Geometry: final body of the model. Coordinates: model frame, mm. A direction names the side the tool comes from. Give positions to 0.01 mm unless a question says otherwise; leave off trailing zeros. Loops run counter-clockwise (first coordinate to the right, second up) from the corner with the lowest first, then second, coordinate; pieces in that order, holes last. Notation, with made-up numbers: (68, 18.25) -> (98, 18.25) arc R17 cw to (98, 36.25) -> close; hole circle Ø9 at (-39.5, -22). An arc over 180 degrees is marked (long way). Answer in a Markdown table with one row per item. Add a question column.
1) Section query C-C (z = 4). Return the cut outline in (x, y).
2) Line query: line 1 (X direction, y = -16, z = 7); line 2 (X direction, y = -22.75, z = 27); line 3 (X direction, y = -2.75, z = 25.25). Output: solid intervals per line, ascending. Write a range as from..to.
3) Access query for faces 1 (the flat face through (-7, -10.414, 15)), 2 (the flat face through (49, -15.038, 15)), 3 (the flat face through (-18.668, -20, 15)), 4 (the flat face through (54, -12.5, 15)). Directions: +Z, -Z, +X, -X, +Y, -Y. A direction counts if a zero-diameter tool reaches every point of the face in a straight line with its end or side. Return the directions, or none.
4) First-contact query: P1, Ø15, axis at x = 24.5, z = 20.5, coming from the +Y side; P2, Ø10, axis at x = -12, z = 25, coming from the -Y side; P3, Ø3, axis at y = -4, z = 16.5, coming from the +X side. Flat tips, straight axial feed; report the tip coordinate or a pass-through.
5) Section query B-B (x = 49.5). Return the cut outline in (y, z).
6) Section query A-A (y = -16.75). Return the cut outline in (x, z).
7) Draft query along X for faces 5 (the flat face through (-28.375, -12, 15)), 6 (the flat face through (60.081, -19, 15)), 7 (the flat face through (5.6, -20, 15)), 8 (the flat face through (-23, 0, 15)). Return one class per face: +X half, -X half, draft (parallel to the pull), parting line (faces both ways), or undercut.
8) Section query D-D (y = -4.25). Return the cut outline in (x, z).
```python
from build123d import *

# Parameters (mm, degrees)
F0_W     = 24.2680183989
F0_H     = 5.0877342001
F0_W_2   = 35.3016227051
F0_H_2   = 3.6045075208
F0_W_3   = 2.852525562
F0_H_3   = 2.53832
F1_DEPTH = 30


with BuildPart() as f1:
    # F0 (on Top) → F1 (new body)
    with BuildSketch(Plane.XY):
        Polygon((-18.6677063226, -10.4143796489), (-18.6677063226, 0), (-28.3749136821, 0), (-28.3749136821, -25), (-18.6677063226, -25), (-18.6677063226, -15.5021138489), align=None)
        with Locations((-6.5336971231, -12.9582467489)):
            Rectangle(F0_W, F0_H)
        Polygon((5.6003120763, 0), (5.6003120763, -10.4143796489), (5.6003120763, -15.5021138489), (5.6003120763, -25), (15.563129677, -25), (15.563129677, -21.3954924792), (15.563129677, 0), align=None)
        with Locations((33.2139410295, -23.1977462396)):
            Rectangle(F0_W_2, F0_H_2)
        Polygon((50.864752382, -21.3954924792), (50.864752382, -25), (60.0811056793, -25), (60.0811056793, -12.5), (50.864752382, -12.5), (50.864752382, -15.03832), align=None)
        with Locations((49.438489601, -13.76916)):
            Rectangle(F0_W_3, F0_H_3)
    extrude(amount=F1_DEPTH)


solid = f1.part
```
Evaluation:
| question | item | result |
|---|---|---|
| 1 | outline | (-28.37, -25) -> (-18.67, -25) -> (-18.67, -15.5) -> (5.6, -15.5) -> (5.6, -25) -> (60.08, -25) -> (60.08, -12.5) -> (48.01, -12.5) -> (48.01, -15.04) -> (50.86, -15.04) -> (50.86, -21.4) -> (15.56, -21.4) -> (15.56, 0) -> (5.6, 0) -> (5.6, -10.41) -> (-18.67, -10.41) -> (-18.67, 0) -> (-28.37, 0) -> close |
| 2 | line 1 | -28.37..-18.67, 5.6..15.56, 50.86..60.08 |
| 2 | line 2 | -28.37..-18.67, 5.6..60.08 |
| 2 | line 3 | -28.37..-18.67, 5.6..15.56 |
| 3 | face 1 | +Z, -Z, +Y |
| 3 | face 2 | +Z, -Z |
| 3 | face 3 | +Z, -Z, -Y |
| 3 | face 4 | +Z, -Z, +X, +Y |
| 4 | P1 | y = -21.4 |
| 4 | P2 | y = -15.5 |
| 4 | P3 | x = 15.56 |
| 5 | outline | (-25, 0) -> (-21.4, 0) -> (-21.4, 30) -> (-25, 30) -> close; (-15.04, 0) -> (-12.5, 0) -> (-12.5, 30) -> (-15.04, 30) -> close |
| 6 | outline | (-28.37, 0) -> (-18.67, 0) -> (-18.67, 30) -> (-28.37, 30) -> close; (5.6, 0) -> (15.56, 0) -> (15.56, 30) -> (5.6, 30) -> close; (50.86, 0) -> (60.08, 0) -> (60.08, 30) -> (50.86, 30) -> close |
| 7 | face 5 | -X half |
| 7 | face 6 | +X half |
| 7 | face 7 | undercut |
| 7 | face 8 | draft |
| 8 | outline | (-28.37, 0) -> (-18.67, 0) -> (-18.67, 30) -> (-28.37, 30) -> close; (5.6, 0) -> (15.56, 0) -> (15.56, 30) -> (5.6, 30) -> close |
